```python
from build123d import *

# Parameters (mm, degrees)
F0_R       = 18.6431523729
F1_DEPTH   = 11.43
F2_R       = 28.8493495365
F3_DEPTH   = 38.1
F4_R       = 18.663241222
F3_FACE1_R = 28.8493495365
F5_DEPTH   = 12.7


with BuildPart() as f1:
    # F0 (on Front) → F1 (new body)
    with BuildSketch(Plane.XZ):
        Circle(F0_R)
    extrude(amount=F1_DEPTH)

    # F2 (on Front) → F3 (join)
    with BuildSketch(Plane.XZ):
        Circle(F2_R)
    extrude(amount=F3_DEPTH)

    # F4 (on face) + F3_face1 (on face) → F5 (cut)
    with BuildSketch(Plane(origin=(0, 0, 0), x_dir=(-1, 0, 0), z_dir=(0, 1, 0))):
        Circle(F4_R)
    with BuildSketch(Plane.XZ.offset(38.1)):
        Circle(F3_FACE1_R)
    extrude(amount=-F5_DEPTH, dir=(0, 1, 0), mode=Mode.SUBTRACT)


solid = f1.part
```
Could you check a few things on this model? Use its own coordinates, in mm. A direction names the side the tool comes from. Round coordinates to 2 decimals unless told otherwise and drop trailing zeros. Loops run counter-clockwise (first coordinate to the right, second up) from the corner with the lowest first, then second, coordinate; pieces in that order, holes last. Notation, with made-up numbers: M 25.5,-0.5 L 71.5,-0.5 A21 ccw 71.5,13.5 Z; hole C -13,72 d3. An arc over 180 degrees is marked long. Put each result on its own line as item: value.
Q1. Thinking about a two-plate mould opening in Z: for faces 1 (the face through (14.81, -6.26, -11.36)), 2 (the face through (0, 0, -19)), 3 (the face through (-6.254, -18.783, -28.163)), which applies, released by +Z, released by -Z, zero draft, split by the parting line, or undercut?
Check result:
face 1: undercut
face 2: zero draft
face 3: split by the parting line
Q2. For pin 1 (18.5 mm diameter, centred on x = 5.5, z = 3, fed in from +Y); pin 2 (2 mm diameter, centred on x = -2.5, y = -23.5, fed in from -Z); pin 3 (5 mm diameter, centred on x = -22, y = -29.5, fed in from +Z), each with a flat end and sliding along its axis, tell me the tip position at first contact or that it passes through.
Check result:
pin 1: y = -12.7
pin 2: z = -28.81
pin 3: z = 21.26
Q3. On a 3-axis mill with a long thin cutter (end or side, diameter ignored), from which of +Z, -Z, +X, -X, +Y, -Y can I reach the whole of each face in a straight line? I mean faces 4 (the face through (0, -12.7, 0)), 5 (the face through (0, -38.1, 0)). Say none if no direction works.
Check result:
face 4: +Y
face 5: +Z, -Z, +X, -X, -Y
Q4. I need wall thicknesses on probe 1 along Z at (x, y) = (0, -3.75); probe 2 along Y at (x, z) = (-17, -2.5); probe 3 along Z at (x, y) = (14.5, -3). Which ranges of each line are inside material? Lowest first, please.
Check result:
probe 1: -28.85 to -18.66, 18.66 to 28.85
probe 2: -38.1 to -12.7
probe 3: -24.94 to -11.75, 11.75 to 24.94
Q5. Imagine slicing it at A-A (z = 0). Write out the boundary of the cut face in (x, y), then the cut area to 3 significant figures.
Check result:
outline: M -28.85,-38.1 L 28.85,-38.1 L 28.85,0 L 18.66,0 L 18.66,-12.7 L -18.66,-12.7 L -18.66,0 L -28.85,0 Z
area: 1,720 mm2
Q6. Imagine slicing it at C-C (y = -5). Write out the boundary of the cut face in (x, z), then the cut area to 3 significant figures.
Check result:
outline: C 0,0 d57.7; hole C 0,0 d37.33
area: 1,520 mm2
Q7. Imagine slicing it at D-D (y = -27.5). Write out the boundary of the cut face in (x, z), then the cut area to 3 significant figures.
Check result:
outline: C 0,0 d57.7
area: 2,610 mm2
Q8. Imagine slicing it at B-B (x = 0). Write out the boundary of the cut face in (y, z).
Check result:
outline: M -38.1,-28.85 L 0,-28.85 L 0,-18.66 L -12.7,-18.66 L -12.7,18.66 L 0,18.66 L 0,28.85 L -38.1,28.85 Z
